Can you work these out from the model? Positions are in its coordinate system, mm. A direction names the side the tool comes from. Round coordinates to 2 decimals unless told otherwise and drop trailing zeros. Loops run counter-clockwise (first coordinate to the right, second up) from the corner with the lowest first, then second, coordinate; pieces in that order, holes last. Notation, with made-up numbers: (7.25, 47) -> (11.25, 47) arc R23 cw to (11.25, 81) -> close; hole circle Ø2 at (68, 59). An arc over 180 degrees is marked (long way). Use a Markdown table: item, result.
from build123d import *

# Parameters (mm, degrees)
MAIN_BODY_W                        = 279.4
MAIN_BODY_H                        = 228.6
MAIN_BODY_EXTRUDE_DEPTH            = 101.6
SKETCH2_W                          = 88.9
SKETCH2_H                          = 215.9
MAIN_BODY_HOLLOW_EXTRUDE_CUT_DEPTH = 273.05
SKETCH3_W                          = 6.35
SKETCH3_H                          = 88.9
SLIDING_DOOR_EXTRUDE_CUT_DEPTH     = 273.05
SKETCH4_W                          = 7.62
SKETCH4_H                          = 25.4
CUT_EXTRUDE3_DEPTH                 = 25.4


with BuildPart() as part:
    # Main Body → Main Body Extrude (new body)
    with BuildSketch(Plane.XY):
        with Locations((60.02161481, -114.3)):
            Rectangle(MAIN_BODY_W, MAIN_BODY_H)
    extrude(amount=MAIN_BODY_EXTRUDE_DEPTH)

    # Sketch2 → Main Body Hollow Extrude Cut (cut)
    with BuildSketch(Plane(origin=(199.72161481, 0, 0), x_dir=(0, 0, -1), z_dir=(1, 0, 0))):
        with Locations((-50.8, -114.3)):
            Rectangle(SKETCH2_W, SKETCH2_H)
    extrude(amount=-MAIN_BODY_HOLLOW_EXTRUDE_CUT_DEPTH, mode=Mode.SUBTRACT)

    # Sketch3 → Sliding Door Extrude Cut (cut)
    with BuildSketch(Plane(origin=(0, 0, 0), x_dir=(1, 0, 0), z_dir=(0, 1, 0))):
        with Locations((190.19661481, -50.8)):
            Rectangle(SKETCH3_W, SKETCH3_H)
    extrude(amount=-SLIDING_DOOR_EXTRUDE_CUT_DEPTH, mode=Mode.SUBTRACT)

    # Sketch4 → Cut-Extrude3 (cut)
    with BuildSketch(Plane.XY.offset(101.6)):
        with Locations((51.13161481, -114.3)):
            Rectangle(SKETCH4_W, SKETCH4_H)
        with Locations((68.91161481, -114.3)):
            Rectangle(SKETCH4_W, SKETCH4_H)
    extrude(amount=-CUT_EXTRUDE3_DEPTH, mode=Mode.SUBTRACT)


solid = part.part
1. Will this pin go through, and if not, where does the flat tip stop? pin 1 Ø8 at (y, z) = (-82, 74.5) entering from +X.
Answer sheet:
| item | result |
|---|---|
| pin 1 | stops at x = -73.33 |
2. I want a section at C-C (y = -96). Please give me the cut outline in (x, z).
Answer sheet:
| item | result |
|---|---|
| outline | (-79.68, 0) -> (199.72, 0) -> (199.72, 6.35) -> (-73.33, 6.35) -> (-73.33, 95.25) -> (199.72, 95.25) -> (199.72, 101.6) -> (-79.68, 101.6) -> close |
3. If we mould it in two halves opening along X, with no side actions, what happens to faces 5 (the flat face through (197, -6.35, 51)), 6 (the flat face through (69, -127, 98)), 7 (the flat face through (199.722, -123, 96)), 8 (the flat face through (193.372, -225, 51))? For each: +X half, -X half, draft (parallel to the pull), parting line (faces both ways), or undercut.
Answer sheet:
| item | result |
|---|---|
| face 5 | draft |
| face 6 | undercut |
| face 7 | +X half |
| face 8 | undercut |
4. Which directions (+Z, -Z, +X, -X, +Y, -Y) give clear straight access to the entire face, cutting with the end or side of a thin tool? Please do faces 1 (the flat face through (59, -222.25, 51)), 2 (the flat face through (-79.678, -116, 50)), 3 (the flat face through (72.722, -114, 98)), 4 (the flat face through (187.022, -225, 51)).
Answer sheet:
| item | result |
|---|---|
| face 1 | +X |
| face 2 | +Z, -Z, -X, +Y, -Y |
| face 3 | +Z |
| face 4 | +Y, -Y |
5. I need wall thicknesses on line 1 (Y direction, x = 85, z = 51); line 2 (Z direction, x = 130, y = -42.5); line 3 (X direction, y = -45, z = 74.5). Which ranges of each line are inside material? Lowest first, please.
Answer sheet:
| item | result |
|---|---|
| line 1 | y = -228.6 to -222.25, -6.35 to 0 |
| line 2 | z = 0 to 6.35, 95.25 to 101.6 |
| line 3 | x = -79.68 to -73.33 |
6. I want a section at A-A (z = 29.5). Please give me the cut outline in (x, y), plus the area to 3 significant figures.
Answer sheet:
| item | result |
|---|---|
| outline | (-79.68, -228.6) -> (187.02, -228.6) -> (187.02, -222.25) -> (-73.33, -222.25) -> (-73.33, -6.35) -> (187.02, -6.35) -> (187.02, 0) -> (-79.68, 0) -> close; (193.37, -228.6) -> (199.72, -228.6) -> (199.72, -222.25) -> (193.37, -222.25) -> close; (193.37, -6.35) -> (199.72, -6.35) -> (199.72, 0) -> (193.37, 0) -> close |
| area | 4,840 mm² |
7. I want a section at B-B (x = 133). Please give me the cut outline in (y, z), plus the area to 3 significant figures.
Answer sheet:
| item | result |
|---|---|
| outline | (-228.6, 0) -> (0, 0) -> (0, 101.6) -> (-228.6, 101.6) -> close; hole (-222.25, 6.35) -> (-6.35, 6.35) -> (-6.35, 95.25) -> (-222.25, 95.25) -> close |
| area | 4,030 mm² |
